Build history of the part. All positions in model axes, mm. Face numbers are marked on the shaded views. A direction names the side the tool comes from. Give positions to 0.01 mm unless a question says otherwise; leave off trailing zeros. Write each loop counter-clockwise with the first axis right and the second up, starting at its lowest first coordinate (ties: lowest second). Pieces come first, ordered by that corner, then holes.
from build123d import *

# Parameters (mm, degrees)
BOX009_W        = 25
BOX009_H        = 20
BOX009_DEPTH    = 8
BOX005_W        = 25
BOX005_H        = 85
BOX005_DEPTH    = 8
BOX002_W        = 75
BOX002_H        = 4
BOX002_DEPTH    = 100
SKETCH001_W     = 25
SKETCH001_H     = 92
POCKET001_DEPTH = 5
FILLET_R        = 5
CHAMFER_SIZE    = 24.99
SKETCH002_W     = 25
SKETCH002_H     = 20
POCKET002_DEPTH = 10
CHAMFER001_SIZE = 5
CHAMFER002_SIZE = 10
POCKET003_DEPTH = 11
POCKET004_DEPTH = 4.5
CHAMFER004_SIZE = 5
BOX008_W        = 25
BOX008_H        = 35
BOX008_DEPTH    = 8
CHAMFER005_SIZE = 5
POCKET006_DEPTH = 8
POCKET007_DEPTH = 5


with BuildPart() as box009:
    # Box009 → Box009 (new body)
    with BuildSketch(Plane(origin=(43, 118, 0), x_dir=(1, 0, 0), z_dir=(0, 0, 1))):
        with Locations((12.5, 10)):
            Rectangle(BOX009_W, BOX009_H)
    extrude(amount=BOX009_DEPTH)


with BuildPart() as box005:
    # Box005 → Box005 (new body)
    with BuildSketch(Plane(origin=(43, 53, 0), x_dir=(1, 0, 0), z_dir=(0, 0, 1))):
        with Locations((12.5, 42.5)):
            Rectangle(BOX005_W, BOX005_H)
    extrude(amount=BOX005_DEPTH)


with BuildPart() as chamfer004:
    # Box002 → Box002 (new body)
    with BuildSketch(Plane(origin=(18, 50, 0), x_dir=(1, 0, 0), z_dir=(0, 0, 1))):
        with Locations((37.5, 2)):
            Rectangle(BOX002_W, BOX002_H)
    extrude(amount=BOX002_DEPTH)

    # Sketch001 → Pocket001 (cut)
    with BuildSketch(Plane(origin=(18, 54, 0), x_dir=(-1, 0, 0), z_dir=(0, 1, 0))):
        with BuildLine():
            Line((-60.4, 93), (-60.4, 70))
            ThreePointArc((-64.6, 70), (-62.5, 67.9), (-60.4, 70))
            Line((-64.6, 70), (-64.6, 93))
            ThreePointArc((-60.4, 93), (-62.5, 95.1), (-64.6, 93))
        make_face()
        with BuildLine():
            Line((-10.4, 93), (-10.4, 70))
            ThreePointArc((-14.6, 70), (-12.5, 67.9), (-10.4, 70))
            Line((-14.6, 70), (-14.6, 93))
            ThreePointArc((-10.4, 93), (-12.5, 95.1), (-14.6, 93))
        make_face()
        with Locations((-37.5, 54)):
            Rectangle(SKETCH001_W, SKETCH001_H)
    extrude(amount=-POCKET001_DEPTH, mode=Mode.SUBTRACT)

    # Fillet
    fillet_edges = [chamfer004.edges().sort_by_distance(p)[0] for p in [
        (93, 52, 100),
        (68, 52, 100),
        (43, 52, 100),
        (18, 52, 100),
    ]]
    fillet(fillet_edges, radius=FILLET_R)

    # Fusion: union Box005
    add(box005.part)

    # Chamfer
    chamfer_edges = [chamfer004.edges().sort_by_distance(p)[0] for p in [
        (43, 54, 4),
        (68, 54, 4),
    ]]
    chamfer(chamfer_edges, length=CHAMFER_SIZE)

    # Sketch002 → Pocket002 (cut)
    with BuildSketch(Plane.XY.offset(8)):
        with Locations((55.5, 60)):
            Rectangle(SKETCH002_W, SKETCH002_H)
    extrude(amount=-POCKET002_DEPTH, mode=Mode.SUBTRACT)

    # Chamfer001
    chamfer001_edges = [chamfer004.edges().sort_by_distance(p)[0] for p in [
        (43, 70, 4),
        (68, 70, 4),
    ]]
    chamfer(chamfer001_edges, length=CHAMFER001_SIZE)

    # Chamfer002
    chamfer002_edges = [chamfer004.edges().sort_by_distance(p)[0] for p in [
        (80.495, 54, 8),
        (30.505, 54, 8),
    ]]
    chamfer(chamfer002_edges, length=CHAMFER002_SIZE)

    # Sketch003 → Pocket003 (cut)
    with BuildSketch(Plane(origin=(0, 0, 0), x_dir=(1, 0, 0), z_dir=(0, 0, -1))):
        with BuildLine():
            Line((57.2, -132), (57.2, -107))
            ThreePointArc((57.2, -107), (55.5, -105.3), (53.8, -107))
            Line((53.8, -107), (53.8, -132))
            ThreePointArc((53.8, -132), (55.5, -133.7), (57.2, -132))
        make_face()
    extrude(amount=-POCKET003_DEPTH, mode=Mode.SUBTRACT)

    # Sketch004 → Pocket004 (cut)
    with BuildSketch(Plane(origin=(0, 0, 0), x_dir=(1, 0, 0), z_dir=(0, 0, -1))):
        with BuildLine():
            Line((51.75, -132), (51.75, -107))
            ThreePointArc((59.25, -107), (55.5, -103.25), (51.75, -107))
            Line((59.25, -107), (59.25, -132))
            ThreePointArc((51.75, -132), (55.5, -135.75), (59.25, -132))
        make_face()
    extrude(amount=-POCKET004_DEPTH, mode=Mode.SUBTRACT)

    # Chamfer004
    chamfer004_edges = [chamfer004.edges().sort_by_distance(p)[0] for p in [
        (43, 138, 4),
        (68, 138, 4),
    ]]
    chamfer(chamfer004_edges, length=CHAMFER004_SIZE)


with BuildPart() as pocket007:
    # Box008 → Box008 (new body)
    with BuildSketch(Plane(origin=(43, 103, 0), x_dir=(1, 0, 0), z_dir=(0, 0, 1))):
        with Locations((12.5, 17.5)):
            Rectangle(BOX008_W, BOX008_H)
    extrude(amount=BOX008_DEPTH)

    # Fusion001: union Chamfer004
    add(chamfer004.part)

    # Cut001: cut Box009
    add(box009.part, mode=Mode.SUBTRACT)

    # Chamfer005
    chamfer005_edges = [pocket007.edges().sort_by_distance(p)[0] for p in [
        (43, 118, 4),
        (68, 118, 4),
    ]]
    chamfer(chamfer005_edges, length=CHAMFER005_SIZE)

    # Sketch006 → Pocket006 (cut)
    with BuildSketch(Plane(origin=(0, 0, 0), x_dir=(1, 0, 0), z_dir=(0, 0, -1))):
        with BuildLine():
            Line((57.25, -85), (57.25, -110))
            ThreePointArc((53.75, -110), (55.5, -111.75), (57.25, -110))
            Line((53.75, -110), (53.75, -85))
            ThreePointArc((57.25, -85), (55.5, -83.25), (53.75, -85))
        make_face()
    extrude(amount=-POCKET006_DEPTH, mode=Mode.SUBTRACT)

    # Sketch007 → Pocket007 (cut)
    with BuildSketch(Plane(origin=(0, 0, 0), x_dir=(1, 0, 0), z_dir=(0, 0, -1))):
        with BuildLine():
            ThreePointArc((59.75, -85.421578), (55.5, -80.729142), (51.25, -85.421578))
            Line((51.25, -85.421578), (51.25, -110))
            ThreePointArc((51.25, -110), (55.5, -114.25), (59.75, -110))
            Line((59.75, -85.421578), (59.75, -110))
        make_face()
    extrude(amount=-POCKET007_DEPTH, mode=Mode.SUBTRACT)


solid = pocket007.part
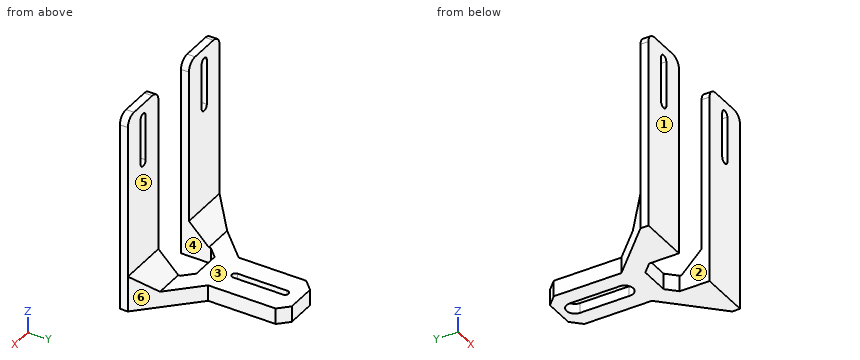
(1) Probe line 1 (X direction, y = 53.5, z = 88); line 2 (Y direction, x = 55.5, z = 2.7); line 3 (X direction, y = 85, z = 1.95). List the from-to ranges inside material, lowest first.
(2) 3-axis set-ups, long thin cutter, end or side, ignore diameter. For the marked faces 1, 2 and 3: which of +Z, -Z, +X, -X, +Y, -Y reach the whole face in a straight line?
(3) Saw through at C-C, the plane x = 80.5. List the corners of the cut face in (y, z).
(4) Saw through at B-B, the plane z = 55.5. List the corners of the cut face in (x, y).
(5) Mould opens along X. For the marked faces 4, 5 and 6 say: +X half, -X half, draft (parallel to the pull), parting line (faces both ways), or undercut.
(6) Saw through at D-D, the plane x = 36. List the corners of the cut face in (y, z), plus the area to 3 significant figures.
(7) Saw through at A-A, the plane y = 56. List the corners of the cut face in (x, z), plus the area to 3 significant figures.
(8) Drop flat-ended pins along their axis: pin 1 (1.5 mm diameter, centred on y = 103.5, z = 3, fed in from -X); pin 2 (5 mm diameter, centred on x = 78, z = 13.5, fed in from +Y); pin 3 (2.5 mm diameter, centred on y = 91.5, z = 1.5, fed in from +X); pin 4 (1 mm diameter, centred on x = 73, y = 77, fed in from -Z). Give the stop position or say it passes through.
Computed values:
1. line 1: x = 18 to 28.4, 32.6 to 43, 68 to 78.4, 82.6 to 93
1. line 2: y = 70 to 80.73, 114.25 to 118
1. line 3: x = 43 to 51.23, 59.77 to 68
2. face 1: +Z, -Z, +X, -X, -Y
2. face 2: +Z, -Z, -Y
2. face 3: +Z, +X, -X, +Y
3. outline: (50, 0) - (66.49, 0) - (66.49, 8) - (64, 8) - (54, 18) - (54, 67.9) - (50, 67.9) - close; (50, 95.1) - (54, 95.1) - (54, 100) - (50, 100) - close
4. outline: (18, 50) - (43, 50) - (43, 54) - (18, 54) - close; (68, 50) - (93, 50) - (93, 54) - (68, 54) - close
5. face 4: undercut
5. face 5: draft
5. face 6: +X half
6. outline: (50, 0) - (71.99, 0) - (71.99, 8) - (64, 8) - (54, 18) - (54, 100) - (50, 100) - close
6. area: 594 mm2
7. outline: (20.01, 0) - (43, 0) - (43, 16) - (20.01, 16) - close; (68, 0) - (90.99, 0) - (90.99, 16) - (68, 16) - close
7. area: 736 mm2
8. pin 1: stops at x = 43
8. pin 2: stops at y = 61
8. pin 3: stops at x = 68
8. pin 4: passes through
